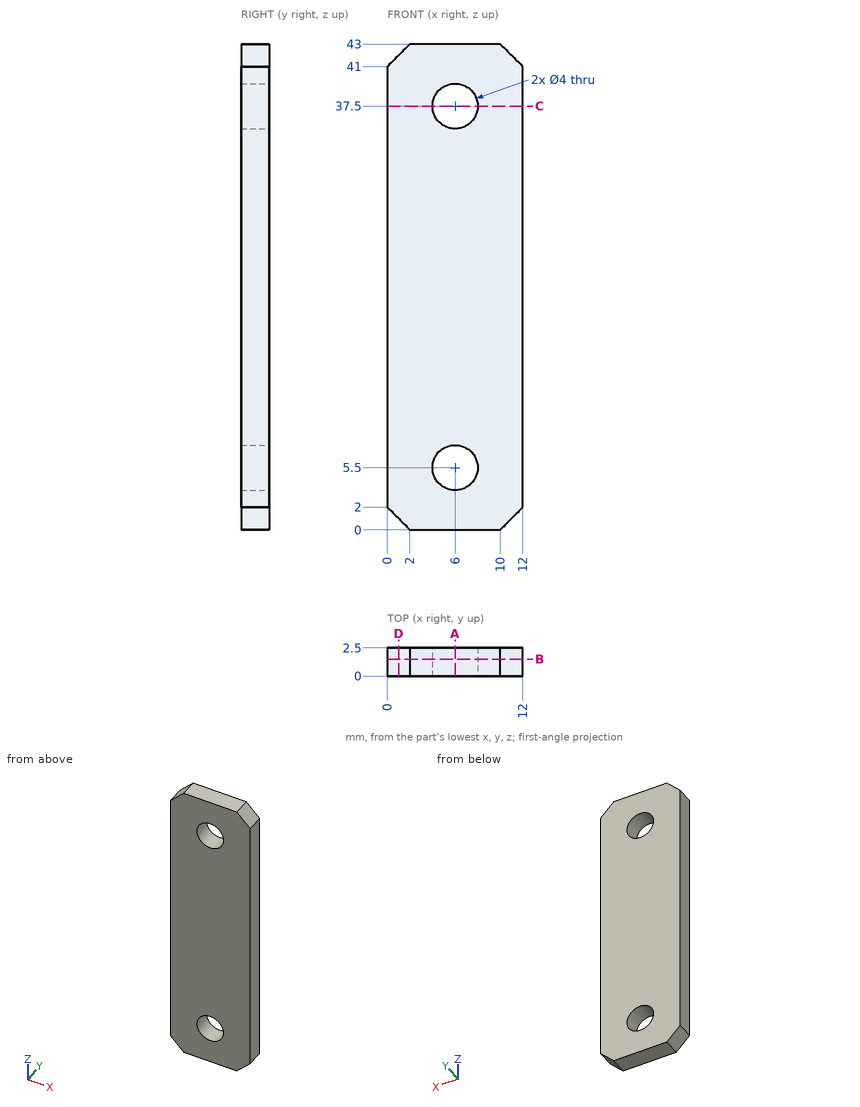
Source: three-view drawing plus pictorial views. Frame: mm from the lowest corner of the part. Round coordinates to 2 decimals unless told otherwise and drop trailing zeros. Write each loop counter-clockwise with the first axis right and the second up, starting at its lowest first coordinate (ties: lowest second). Pieces come first, ordered by that corner, then holes. Notation, with made-up numbers: M 30,33.5 L 58,33.5 A18 cw 58,51.5 Z; hole C 81.5,41.5 d9. An arc over 180 degrees is marked long. Write item = value, one per line.
Item 1: Section query A-A on x = 6. Return loops of the section in (y, z), then the cut area to 3 significant figures.
Findings:
outline = M 0,0 L 2.5,0 L 2.5,3.5 L 0,3.5 Z; M 0,7.5 L 2.5,7.5 L 2.5,35.5 L 0,35.5 Z; M 0,39.5 L 2.5,39.5 L 2.5,43 L 0,43 Z
area = 87.5 mm^2
Item 2: Material intervals for line 1 along Z through (x, y) = (6, 0.7); line 2 along X through (y, z) = (1.9, 5.5); line 3 along Z through (x, y) = (4.75, 2), sorted ascending. Write a range as [from, to].
Findings:
line_1 = [0, 3.5], [7.5, 35.5], [39.5, 43]
line_2 = [0, 4], [8, 12]
line_3 = [0, 3.94], [7.06, 35.94], [39.06, 43]
Item 3: Section query B-B on y = 1.5. Return loops of the section in (x, z).
Findings:
outline = M 0,2 L 2,0 L 10,0 L 12,2 L 12,41 L 10,43 L 2,43 L 0,41 Z; hole C 6,5.5 d4; hole C 6,37.5 d4
Item 4: Section query D-D on x = 1. Return loops of the section in (y, z), then the cut area to 4 significant figures.
Findings:
outline = M 0,1 L 2.5,1 L 2.5,42 L 0,42 Z
area = 102.5 mm^2
Item 5: Section query C-C on z = 37.5. Return loops of the section in (x, y).
Findings:
outline = M 0,0 L 4,0 L 4,2.5 L 0,2.5 Z; M 8,0 L 12,0 L 12,2.5 L 8,2.5 Z
